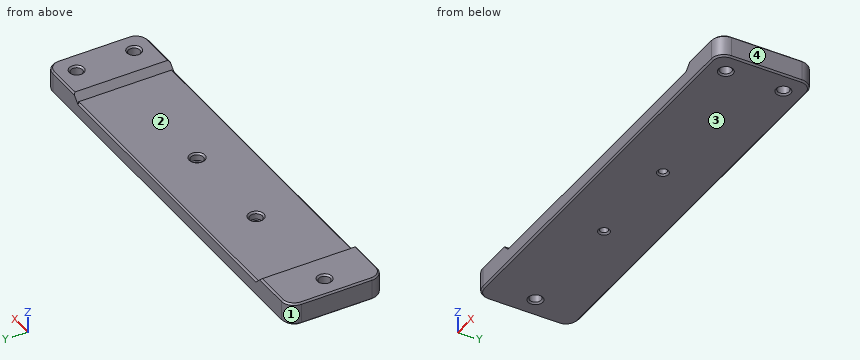
Autodesk Inventor part; units mm, degrees
ref_plane "YZ Plane" through (0, 0, 0) normal (1, 0, 0) x (0, 1, 0)
ref_plane "XZ Plane" through (0, 0, 0) normal (0, 1, 0) x (-1, 0, 0)
ref_plane "XY Plane" through (0, 0, 0) normal (0, 0, 1) x (1, 0, 0)
sketch "Sketch1" plane through (0, 0, 0) normal (0, 0, 1) x (1, 0, 0)
  line L0 (-65, 15) -> (65, 15)
  line L1 (65, 15) -> (65, -15)
  line L2 (65, -15) -> (-65, -15)
  line L3 (-65, -15) -> (-65, 15)
  point P0 (0, 0)
  point P1 (0, 15)
  point P2 (65, 0)
  dimension "d0" = 130
  dimension "d1" = 30
extrude "Extrusion1" add sketch "Sketch1" along normal blind 7
sketch "Sketch2" plane through (0, 0, 7) normal (0, 0, 1) x (1, 0, 0)
  line L0 (58.5, 9) -> (58.5, -9) construction
  line L1 (-58.5, 0) -> (58.5, 0) construction
  point P0 (0, 0)
  point P1 (0, 0)
  dimension "d4" = 117
  dimension "d5" = 18
hole "Hole1" at (-58.5, 0, 7) at (58.5, 9, 7) at (58.5, -9, 7) direction (0, 0, -1) diameter 3.6 end through all
sketch "Sketch3" plane through (0, 0, 7) normal (0, 0, 1) x (1, 0, 0)
  line L0 (65, 15) -> (-65, 15)
  line L1 (-65, -15) -> (65, -15)
  line L2 (-50, 15) -> (50, 15)
  line L3 (50, 15) -> (50, -15)
  line L4 (50, -15) -> (-50, -15)
  line L5 (-50, -15) -> (-50, 15)
  point P0 (0, 0)
  point P1 (0, -15)
  dimension "d13" = 100
extrude "Extrusion2" cut sketch "Sketch3" against normal blind 2
sketch "Sketch4" plane through (0, 0, 5) normal (0, 0, 1) x (1, 0, 0)
  line L0 (-21.9201, 0) -> (9.5799, 0) construction
  point P0 (0, 0)
  dimension "d16" = 31.5
hole "Hole2" at (-21.9201, 0, 5) at (9.5799, 0, 5) direction (0, 0, -1) diameter 2.5 end through all counterbore diameter 3.9 counterbore depth 2.3
fillet "Fillet1" radius 4 4 edges at (-65, -15, 3.5) (-65, 15, 3.5) (65, 15, 3.5) (65, -15, 3.5)
chamfer "Chamfer1" distance 2 angle 45 2 edges at (-50, 0, 5) (50, 0, 5)
chamfer "Chamfer2" distance 0.5 angle 45 10 edges at (-21.9201, 1.95, 5) (9.5799, 1.95, 5) (58.5, -7.2, 7) (58.5, 10.8, 7) (-58.5, 1.8, 7) (58.5, -7.2, 0) (-58.5, 1.8, 0) (58.5, 10.8, 0) (-21.9201, 1.25, 0) (9.5799, 1.25, 0)
chamfer "Chamfer3" distance 0.5 angle 45 20 edges at (0, 15, 5) (-55.5, 15, 7) (-63.8284, 13.8284, 7) (-65, 0, 7) (-63.8284, -13.8284, 7) (-55.5, -15, 7) (0, -15, 5) (55.5, 15, 7) (63.8284, 13.8284, 7) (65, 0, 7) (63.8284, -13.8284, 7) (55.5, -15, 7) (0, 15, 0) (-63.8284, 13.8284, 0) (-65, 0, 0) (-63.8284, -13.8284, 0) (0, -15, 0) (63.8284, -13.8284, 0) (65, 0, 0) (63.8284, 13.8284, 0)
properties part number "LRS-150-din-bracket" material "ABS Plastic"
Geometry: final body of the model. Coordinates: model frame, mm. Face numbers are marked on the shaded views. Give positions to 0.01 mm unless a question says otherwise; leave off trailing zeros. Loops run counter-clockwise (first coordinate to the right, second up) from the corner with the lowest first, then second, coordinate; pieces in that order, holes last. Notation, with made-up numbers: (-34.5, -39.75) -> (-15.5, -39.75) arc R26 ccw to (-15.5, -19.75) -> close; hole circle Ø6 at (22.25, 59). An arc over 180 degrees is marked (long way). Use CSV: the item, a comma, the result in double quotes.
(1) First-contact query: P1, Ø4.5, axis at x = -21.5, y = 0.5, coming from the +Z side; P2, Ø4.5, axis at x = 58.5, y = 9, coming from the -Z side; P3, Ø3, axis at x = -21.92, y = 0, coming from the -Z side; P4, Ø4, axis at x = 5.5, z = 5, coming from the -Y side. Flat tips, straight axial feed; report the tip coordinate or a pass-through.
From the geometry:
P1,"z = 5"
P2,"z = 0.05"
P3,"z = 0.25"
P4,"y = -15"
(2) Pull-direction query (X, two-part tool) for the marked faces 1, 2, 3 and 4; classes: released by +X, released by -X, zero draft, split by the parting line, or undercut.
From the geometry:
face 1,"released by -X"
face 2,"undercut"
face 3,"zero draft"
face 4,"released by +X"
(3) Cut plane D-D (x = -18). Output: boundary loops of the cut face in (y, z), plus the area to 4 significant figures.
From the geometry:
outline,"(-15, 0.5) -> (-14.5, 0) -> (14.5, 0) -> (15, 0.5) -> (15, 4.5) -> (14.5, 5) -> (-14.5, 5) -> (-15, 4.5) -> close"
area,"149.5 mm^2"
(4) Ray query, line 1 along X through (y, z) = (0, 1.75); line 2 along X through (y, z) = (0, 4.05); line 3 along Y through (x, z) = (58.5, 3.65). Return the intervals inside material, ascending. Write a range as [from, to].
From the geometry:
line 1,"[-65, -60.3], [-56.7, -23.17], [-20.67, 8.33], [10.83, 65]"
line 2,"[-65, -60.3], [-56.7, -23.87], [-19.97, 7.63], [11.53, 65]"
line 3,"[-15, -10.8], [-7.2, 7.2], [10.8, 15]"
(5) Cut plane B-B (x = 58.5). Output: boundary loops of the cut face in (y, z).
From the geometry:
outline,"(-15, 0.5) -> (-14.5, 0) -> (-11.3, 0) -> (-10.8, 0.5) -> (-10.8, 6.5) -> (-11.3, 7) -> (-14.5, 7) -> (-15, 6.5) -> close; (-7.2, 0.5) -> (-6.7, 0) -> (6.7, 0) -> (7.2, 0.5) -> (7.2, 6.5) -> (6.7, 7) -> (-6.7, 7) -> (-7.2, 6.5) -> close; (10.8, 0.5) -> (11.3, 0) -> (14.5, 0) -> (15, 0.5) -> (15, 6.5) -> (14.5, 7) -> (11.3, 7) -> (10.8, 6.5) -> close"
